The drawing under review shows one solid part. Ordinate dimensions are in mm from its lowest x, y, z. Coordinates: 2 decimals unless noted, no trailing zeros. Order: outer loops, then holes, each group sorted by start corner. A loop starts at its lowest first (then second) coordinate and runs counter-clockwise, first axis right, second up. Notation, with made-up numbers: (25.5, 48) -> (49.5, 48) arc R20 cw to (49.5, 54) -> close; hole circle Ø8 at (-23, -13). An arc over 180 degrees is marked (long way). Put each result on its own line as item: value.
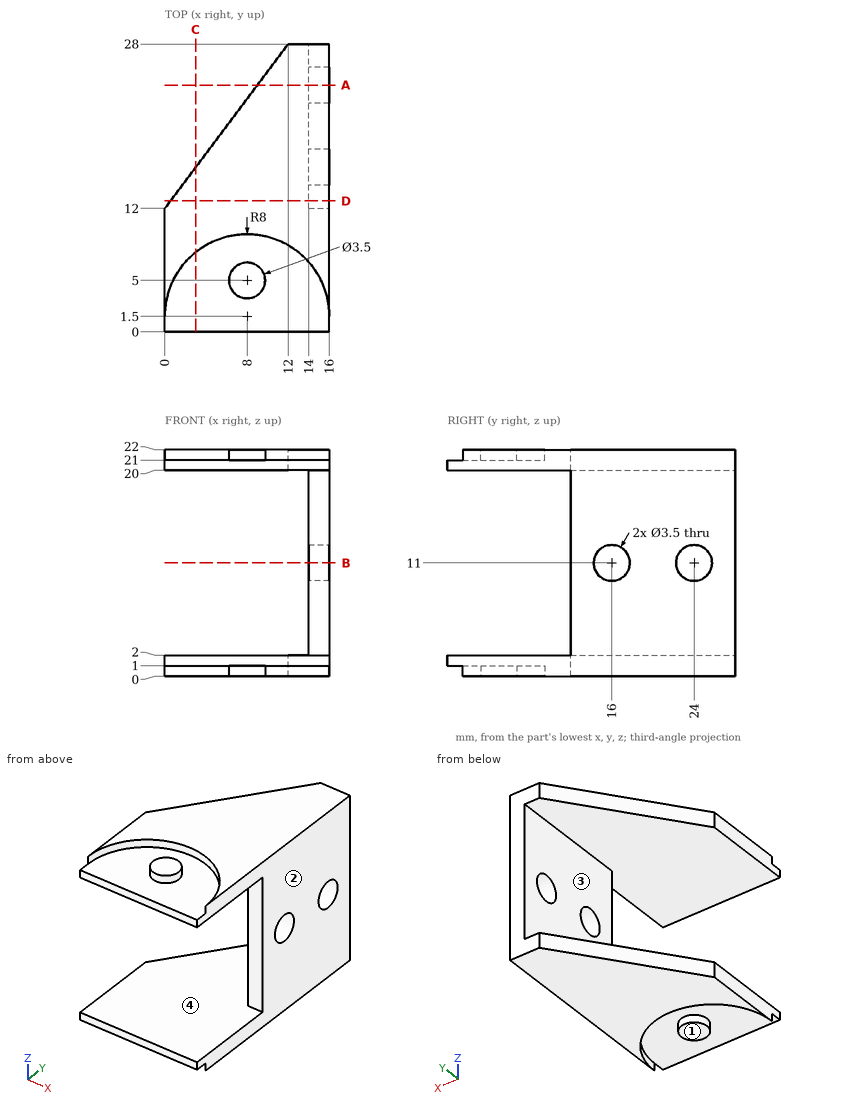
Item 1: Consider section C-C on x = 3. Write out the cut boundary in (y, z) (3 decimals).
Answers below:
outline: (0, 1) -> (7.745, 1) -> (7.745, 0) -> (16, 0) -> (16, 2) -> (0, 2) -> close; (0, 20) -> (16, 20) -> (16, 22) -> (7.745, 22) -> (7.745, 21) -> (0, 21) -> close
Item 2: Consider section A-A on y = 24. Write out the cut boundary in (x, z).
Answers below:
outline: (9, 0) -> (16, 0) -> (16, 9.25) -> (14, 9.25) -> (14, 2) -> (9, 2) -> close; (9, 20) -> (14, 20) -> (14, 12.75) -> (16, 12.75) -> (16, 22) -> (9, 22) -> close
Item 3: Mouldability with a two-part tool opening along Z and no side actions: class the marked faces 1, 2, 3 and 4 as +Z half, -Z half, draft (parallel to the pull), parting line (faces both ways), or undercut.
Answers below:
face 1: -Z half
face 2: draft
face 3: undercut
face 4: undercut
Item 4: Consider section B-B on z = 11. Write out the cut boundary in (x, y).
Answers below:
outline: (14, 12) -> (16, 12) -> (16, 14.25) -> (14, 14.25) -> close; (14, 17.75) -> (16, 17.75) -> (16, 22.25) -> (14, 22.25) -> close; (14, 25.75) -> (16, 25.75) -> (16, 28) -> (14, 28) -> close
Item 5: For pin 1 Ø7.5 at (x, y) = (5.5, 4) entering from -Z; pin 2 Ø8 at (y, z) = (21, 9) entering from -X; pin 3 Ø6 at (x, z) = (11.5, 9.5) entering from -Y; pin 4 Ø3 at (y, z) = (16, 11) entering from +X, all flat-tipped, find the tip position at first contact; note any pin that passes through.
Answers below:
pin 1: z = 0
pin 2: x = 14
pin 3: y = 12
pin 4: through
Item 6: For line 1 (Y direction, x = 14.75, z = 11); line 2 (Z direction, x = 8, y = 15); line 3 (Z direction, x = 14.45, y = 16), list the stretches that pass through material, from the lowest coordinate up. Write a range as from..to.
Answers below:
line 1: 12..14.25, 17.75..22.25, 25.75..28
line 2: 0..2, 20..22
line 3: 0..9.25, 12.75..22
Item 7: Consider section D-D on y = 12.75. Write out the cut boundary in (x, z).
Answers below:
outline: (0.56, 0) -> (16, 0) -> (16, 22) -> (0.56, 22) -> (0.56, 20) -> (14, 20) -> (14, 2) -> (0.56, 2) -> close
